For this review, take the finished solid that the model builds, in its own axes (mm). Coordinates: 2 decimals unless noted, no trailing zeros. Loops run counter-clockwise (first coordinate to the right, second up) from the corner with the lowest first, then second, coordinate; pieces in that order, holes last. Notation, with made-up numbers: (47, -24) - (72, -24) arc R11 ccw to (72, -19) - close; hole circle Ø5 at (-38, 26). An arc over 180 degrees is marked (long way). One line per item, written item: value. Start each with the question number.
1. Take a section at C-C, the plane y = -20.5. State the section outline as (x, z) points.
2. Take a section at B-B, the plane z = 2.5. State the section outline as (x, y) points, and give its area (3 significant figures).
3. Take a section at D-D, the plane x = 50. State the section outline as (y, z) points.
4. Take a section at A-A, the plane x = 28. State the section outline as (y, z) points, and give its area (3 significant figures).
5. To check wall thickness, follow line 1 (X direction, y = -9.5, z = 0.7); line 2 (X direction, y = -13, z = 0.45); line 3 (Y direction, x = 49.5, z = 2.5). State the ranges of each line that lie inside material, in increasing order. Write a range as from..to.
```python
from build123d import *

# Parameters (mm, degrees)
BOSS_EXTRUDE1_DEPTH = 3
SKETCH2_R           = 1.5
CUT_EXTRUDE1_DEPTH  = 3
CUT_EXTRUDE2_DEPTH  = 3


with BuildPart() as part:
    # Sketch1 → Boss-Extrude1 (new body)
    with BuildSketch(Plane.XY):
        with BuildLine():
            Line((-52.51020312, -2.31327399), (47.128491464, 3.68672601))
            ThreePointArc((47.128491464, 3.68672601), (64.120955569, -12.31327399), (47.128491464, -28.31327399))
            Line((47.128491464, -28.31327399), (-52.51020312, -22.31327399))
            ThreePointArc((-52.51020312, -22.31327399), (-61.926141798, -12.31327399), (-52.51020312, -2.31327399))
        make_face()
    extrude(amount=BOSS_EXTRUDE1_DEPTH)

    # Sketch2 → Cut-Extrude1 (cut)
    with BuildSketch(Plane.XY.offset(3)):
        with Locations((12.091972574, -12.31327399)):
            Circle(SKETCH2_R)
        with Locations((-15.908027426, -12.31327399)):
            Circle(SKETCH2_R)
        with Locations((-51.908027426, -12.31327399)):
            Circle(SKETCH2_R)
        with BuildLine():
            Line((18.75680016, -8.728910804), (47.50542085, -6.040638414))
            ThreePointArc((47.50542085, -6.040638414), (54.391972574, -12.31327399), (47.50542085, -18.585909567))
            Line((47.50542085, -18.585909567), (18.75680016, -15.897637177))
            ThreePointArc((18.75680016, -15.897637177), (15.491972574, -12.31327399), (18.75680016, -8.728910804))
        make_face()
    extrude(amount=-CUT_EXTRUDE1_DEPTH, mode=Mode.SUBTRACT)

    # Sketch3 → Cut-Extrude2 (cut)
    with BuildSketch(Plane(origin=(0, 0, 0), x_dir=(-1, 0, 0), z_dir=(0, 0, -1))):
        with BuildLine():
            Line((16.640273069, -0.15327399), (68.701590892, -0.15327399))
            Line((68.701590892, -0.15327399), (68.701590892, -19.932639697))
            Line((68.701590892, -19.932639697), (68.701590892, -24.47327399))
            Line((68.701590892, -24.47327399), (16.640273069, -24.47327399))
            ThreePointArc((16.640273069, -24.47327399), (28.090054502, -12.31327399), (16.640273069, -0.15327399))
        make_face()
    extrude(amount=-CUT_EXTRUDE2_DEPTH, mode=Mode.SUBTRACT)


solid = part.part
```
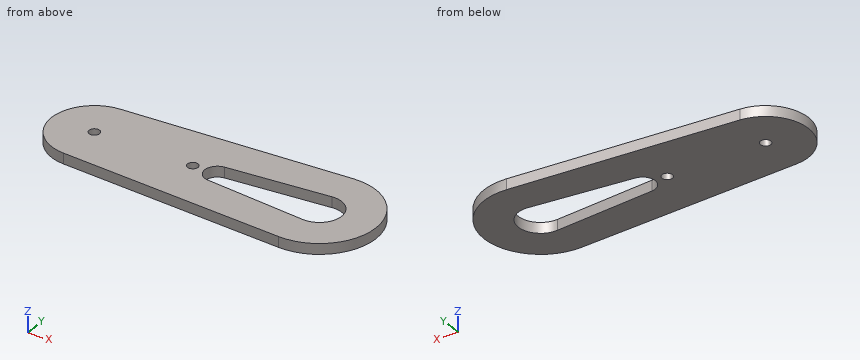
Solutions:
1. outline: (-24.93, 0) - (61.87, 0) - (61.87, 3) - (-24.93, 3) - close
2. outline: (-16.64, -24.47) - (47.13, -28.31) arc R16.03 ccw (long way) to (47.13, 3.69) - (-16.64, -0.15) arc R12.18 ccw to start; hole circle Ø3 at (-15.91, -12.31); hole circle Ø3 at (12.09, -12.31); hole (18.76, -15.9) - (47.51, -18.59) arc R6.3 ccw (long way) to (47.51, -6.04) - (18.76, -8.73) arc R3.6 ccw to start
2. area: 2,060 mm2
3. outline: (-28.23, 0) - (-18.32, 0) - (-18.32, 3) - (-28.23, 3) - close; (-6.31, 0) - (3.6, 0) - (3.6, 3) - (-6.31, 3) - close
4. outline: (-27.16, 0) - (-16.76, 0) - (-16.76, 3) - (-27.16, 3) - close; (-7.86, 0) - (2.53, 0) - (2.53, 3) - (-7.86, 3) - close
4. area: 62.4 mm2
5. line 1: -27.76..16.85, 53.73..63.87
5. line 2: -28.07..-17.24, -14.57..10.76, 13.43..15.56, 54.35..64.11
5. line 3: -28.28..-18.45, -6.17..3.65
